Source: CAD feature listing. Evaluate the final solid. Frame: model axes, mm. A direction names the side the tool comes from. Round coordinates to 2 decimals unless told otherwise and drop trailing zeros. Loops run counter-clockwise (first coordinate to the right, second up) from the corner with the lowest first, then second, coordinate; pieces in that order, holes last.
Item 1: Access query for faces 4 (the conical face through (-87.451, 162.082, 8.938)), 5 (the flat face through (-125.536, 84.09, 2.465)), 6 (the flat face through (-37, 86, 5)), 7 (the flat face through (-37, 160, 49)). Directions: +Z, -Z, +X, -X, +Y, -Y. A direction counts if a zero-diameter tool reaches every point of the face in a straight line with its end or side. Return the directions, or none.
Item 2: Ray query, L1, parallel to Y at x = -66, z = 8; L2, parallel to X at y = 15, z = 27; L3, parallel to X at y = 163.5, z = 26.5. Return the intervals inside material, ascending.
Item 3: First-contact query: P1, Ø7, axis at x = -131, y = 88.5, coming from the +Z side; P2, Ø2.5, axis at y = 107.5, z = 3.5, coming from the -X side; P3, Ø8, axis at x = -45.5, z = 20, coming from the -Y side. Flat tips, straight axial feed; report the tip coordinate or a pass-through.
Item 4: Section query C-C on y = 155.5. Return loops of the section in (x, z), then the cut area to 3 significant figures.
Item 5: Section query A-A on y = 103. Return loops of the section in (x, z), then the cut area to 3 significant figures.
Item 6: Section query B-B on z = 40. Give the number of separate pieces and of enclosed holes in the cut face, then the cut area to 3 significant figures.
Item 7: Pull-direction query (X, two-part tool) for faces 1 (the flat face through (-137.03, 160.14, 24.16)), 2 (the flat face through (-39, 84, 2)), 3 (the flat face through (-128, 86, 5)); classes: released by +X, released by -X, zero draft, split by the parting line, or undercut.
```python
from build123d import *

# Parameters (mm, degrees)
BOX004_W                = 40
BOX004_H                = 20
BOX004_DEPTH            = 49
BOX004_PLACEMENT_ANGLE  = 257.9
BOX003_W                = 40
BOX003_H                = 20
BOX003_DEPTH            = 49
BOX003_PLACEMENT_ANGLE  = 282.8
BOX001_W                = 105.5
BOX001_H                = 20
BOX001_DEPTH            = 49
BOX007_W                = 5
BOX007_H                = 135
BOX007_DEPTH            = 5
BOX007_PLACEMENT_ANGLE  = 352.25
BOX008_W                = 5
BOX008_H                = 130
BOX008_DEPTH            = 5
CONE001_ROLL_ANGLE      = 89.4112
CONE001_PITCH_ANGLE     = 3.998897
CONE001_PLACEMENT_ANGLE = 0.893236
BOX002_W                = 40
BOX002_H                = 20
BOX002_DEPTH            = 49
BOX002_PLACEMENT_ANGLE  = 76
BOX005_W                = 40
BOX005_H                = 20
BOX005_DEPTH            = 49
BOX005_PLACEMENT_ANGLE  = 95
BOX_W                   = 89
BOX_H                   = 20
BOX_DEPTH               = 49


with BuildPart() as cube004:
    # Box004 → Box004 (new body)
    with BuildSketch(Plane.XY):
        with Locations((20, 10)):
            Rectangle(BOX004_W, BOX004_H)
    extrude(amount=BOX004_DEPTH)


with BuildPart() as cube004_1:
    # Box004 placement: moved
    add(cube004.part.moved(Location((-152.64395, 182.723164, 0))).rotate(Axis((-152.64395, 182.723164, 0), (0, 0, 1)), BOX004_PLACEMENT_ANGLE))


with BuildPart() as cone:
    # Cone → Cone (revolve)
    with BuildSketch(Plane(origin=(-86.5, 170, 57.03), x_dir=(1, 0, 0), z_dir=(0, 0, -1))):
        Polygon((0, 0), (46.38, 0), (50.75, 20.1), (0, 20.1), align=None)
    revolve(axis=Axis((-86.5, 170, 57.03), (0, -1, 0)))


with BuildPart() as cube003:
    # Box003 → Box003 (new body)
    with BuildSketch(Plane.XY):
        with Locations((20, 10)):
            Rectangle(BOX003_W, BOX003_H)
    extrude(amount=BOX003_DEPTH)


with BuildPart() as cube003_1:
    # Box003 placement: moved
    add(cube003.part.moved(Location((-38.594683, 170.816256, 0))).rotate(Axis((-38.594683, 170.816256, 0), (0, 0, 1)), BOX003_PLACEMENT_ANGLE))


with BuildPart() as cut003:
    # Box001 → Box001 (new body)
    with BuildSketch(Plane(origin=(-139.5, 150, 0), x_dir=(1, 0, 0), z_dir=(0, 0, 1))):
        with Locations((52.75, 10)):
            Rectangle(BOX001_W, BOX001_H)
    extrude(amount=BOX001_DEPTH)

    # Cut003: cut Cube003
    add(cube003_1.part, mode=Mode.SUBTRACT)


with BuildPart() as cut005:
    # Box007 → Box007 (new body)
    with BuildSketch(Plane.XY):
        with Locations((2.5, 67.5)):
            Rectangle(BOX007_W, BOX007_H)
    extrude(amount=BOX007_DEPTH)


with BuildPart() as cut005_1:
    # Box007 placement: moved
    add(cut005.part.moved(Location((-121.333055, 16.130182, 0))).rotate(Axis((-121.333055, 16.130182, 0), (0, 0, -1)), BOX007_PLACEMENT_ANGLE))

    # Fusion: union Cut003
    add(cut003.part)

    # Cut004: cut Cone
    add(cone.part, mode=Mode.SUBTRACT)

    # Cut005: cut Cube004
    add(cube004_1.part, mode=Mode.SUBTRACT)


with BuildPart() as cube008:
    # Box008 → Box008 (new body)
    with BuildSketch(Plane(origin=(-39, 20, 0), x_dir=(1, 0, 0), z_dir=(0, 0, 1))):
        with Locations((2.5, 65)):
            Rectangle(BOX008_W, BOX008_H)
    extrude(amount=BOX008_DEPTH)


with BuildPart() as cone002:
    # Cone002 → Cone002 (revolve)
    with BuildSketch(Plane(origin=(-77.8, 20.1, 57.03), x_dir=(1, 0, 0), z_dir=(0, 0, -1))):
        Polygon((0, 0), (42.5, 0), (39.25, 20.1), (0, 20.1), align=None)
    revolve(axis=Axis((-77.8, 20.1, 57.03), (0, -1, 0)))


with BuildPart() as cone001:
    # Cone001 → Cone001 (revolve)
    with BuildSketch(Plane.XZ):
        Polygon((0, 0), (41.5, 0), (39.25, 25), (0, 25), align=None)
    revolve(axis=Axis((0, 0, 0), (0, 0, 1)))


with BuildPart() as cone001_1:
    # Cone001 roll: moved
    add(cone001.part.rotate(Axis((0, 0, 0), (1, 0, 0)), CONE001_ROLL_ANGLE))


with BuildPart() as cone001_2:
    # Cone001 pitch: moved
    add(cone001_1.part.rotate(Axis((0, 0, 0), (0, 1, 0)), CONE001_PITCH_ANGLE))


with BuildPart() as cone001_3:
    # Cone001 placement: moved
    add(cone001_2.part.moved(Location((-77.76807, 22.976255, 59.052418))).rotate(Axis((-77.76807, 22.976255, 59.052418), (0, 0, 1)), CONE001_PLACEMENT_ANGLE))


with BuildPart() as cube002:
    # Box002 → Box002 (new body)
    with BuildSketch(Plane.XY):
        with Locations((20, 10)):
            Rectangle(BOX002_W, BOX002_H)
    extrude(amount=BOX002_DEPTH)


with BuildPart() as cube002_1:
    # Box002 placement: moved
    add(cube002.part.moved(Location((-143.09, 17.91, 0))).rotate(Axis((-143.09, 17.91, 0), (0, 0, -1)), BOX002_PLACEMENT_ANGLE))


with BuildPart() as cube005:
    # Box005 → Box005 (new body)
    with BuildSketch(Plane.XY):
        with Locations((20, 10)):
            Rectangle(BOX005_W, BOX005_H)
    extrude(amount=BOX005_DEPTH)


with BuildPart() as cube005_1:
    # Box005 placement: moved
    add(cube005.part.moved(Location((-33.959196, 21.508677, 0))).rotate(Axis((-33.959196, 21.508677, 0), (0, 0, -1)), BOX005_PLACEMENT_ANGLE))


with BuildPart() as fusion001:
    # Box → Box (new body)
    with BuildSketch(Plane(origin=(-123, 0, 0), x_dir=(1, 0, 0), z_dir=(0, 0, 1))):
        with Locations((44.5, 10)):
            Rectangle(BOX_W, BOX_H)
    extrude(amount=BOX_DEPTH)

    # Cut: cut Cube005
    add(cube005_1.part, mode=Mode.SUBTRACT)

    # Cut001: cut Cube002
    add(cube002_1.part, mode=Mode.SUBTRACT)

    # Cut002: cut Cone001
    add(cone001_3.part, mode=Mode.SUBTRACT)

    # Cut006: cut Cone002
    add(cone002.part, mode=Mode.SUBTRACT)

    # Fusion001: union Cut005, Cube008
    add(cut005_1.part)
    add(cube008.part)


solid = fusion001.part
```
Data:
1. face 4: +Z
1. face 5: +Z, -Z
1. face 6: +Z, +X, -X
1. face 7: +Z, +X, -X, +Y, -Y
2. L1: y = 0 to 20, 150 to 170
2. L2: x = -121.75 to -106.7, -48.9 to -34.53
2. L3: x = -136.31 to -123.27, -49.73 to -36.93
3. P1: stops at z = 5
3. P2: stops at x = -133.94
3. P3: stops at y = 0
4. outline: (-138.03, 0) - (-35.11, 0) - (-35.11, 49) - (-37.62, 49) arc R49.53 cw to (-135.38, 49) - (-138.03, 49) - close
4. area: 1,980 mm2
5. outline: (-133.16, 0) - (-128.11, 0) - (-128.11, 5) - (-133.16, 5) - close; (-39, 0) - (-34, 0) - (-34, 5) - (-39, 5) - close
5. area: 50.2 mm2
6. separate pieces: 4
6. enclosed holes: 0
6. area: 425 mm2
7. face 1: released by -X
7. face 2: undercut
7. face 3: zero draft
